Read the model definition and answer for the solid it produces. Units are mm, in the model's axes. Coordinates: 2 decimals unless noted, no trailing zeros. Write each loop counter-clockwise with the first axis right and the second up, starting at its lowest first coordinate (ties: lowest second). Pieces come first, ordered by that corner, then holes.
(1) The part is cut by section A-A, the plane x = -70. Determine the outline of the cut face in (y, z), and give its area (3 significant figures).
(2) Given pin 1 (9.5 mm diameter, centred on x = 0.5, y = 17, fed in from -Z); pin 2 (4 mm diameter, centred on y = 26, z = -8.5, fed in from -X); pin 3 (3.5 mm diameter, centred on x = -344.5, y = 13.5, fed in from -Z); pin 4 (5 mm diameter, centred on y = 12, z = 22.5, fed in from +X), each flat-ended and moving along its own axis, determine where each tip first touches the part or whether it passes through.
(3) Straight lines are drawn through the part: line 1 along X through (y, z) = (15, -12.5); line 2 along X through (y, z) = (15, -14); line 3 along Y through (x, z) = (345, -17). For each, find the intervals that lie inside material, in ascending order.
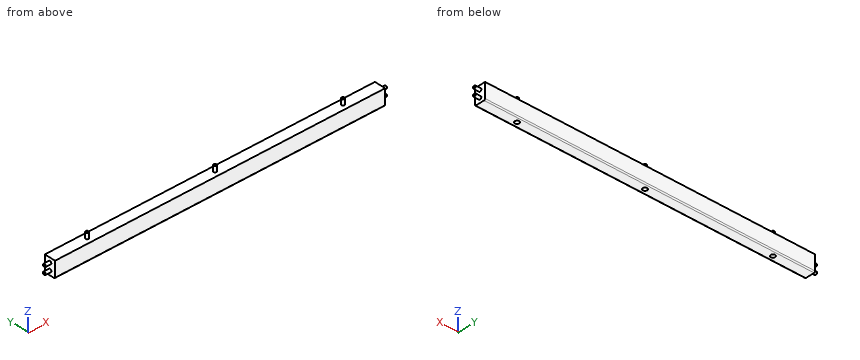
```python
from build123d import *

# Parameters (mm, degrees)
F0_W      = 890
F0_H      = 43
F1_DEPTH  = 30
F2_R      = 4
F3_DEPTH  = 16
F4_SIZE   = 1
F5_R      = 4
F6_DEPTH  = 16
F7_SIZE   = 1
F8_R      = 3
F9_R      = 6
F10_DEPTH = 16
F11_R     = 4
F12_DEPTH = 16
F13_SIZE  = 1


with BuildPart() as f1:
    # F0 (on Front) → F1 (new body)
    with BuildSketch(Plane.XZ):
        Rectangle(F0_W, F0_H)
    extrude(amount=-F1_DEPTH)

    # F2 (on face) → F3 (join)
    with BuildSketch(Plane.YZ.offset(445)):
        with Locations((15, 9.5)):
            Circle(F2_R)
        with Locations((15, -9.5)):
            Circle(F2_R)
    extrude(amount=F3_DEPTH)

    # F4
    f4_edges = [f1.edges().sort_by_distance(p)[0] for p in [
        (461, 11, 9.5),
        (461, 11, -9.5),
    ]]
    chamfer(f4_edges, length=F4_SIZE)

    # F5 (on face) → F6 (join)
    with BuildSketch(Plane(origin=(-445, 0, 0), x_dir=(0, -1, 0), z_dir=(-1, 0, 0))):
        with Locations((-15, 9.5)):
            Circle(F5_R)
        with Locations((-15, -9.5)):
            Circle(F5_R)
    extrude(amount=F6_DEPTH)

    # F7
    f7_edges = [f1.edges().sort_by_distance(p)[0] for p in [
        (-461, 19, 9.5),
        (-461, 19, -9.5),
    ]]
    chamfer(f7_edges, length=F7_SIZE)

    # F8
    f8_edges = [f1.edges().sort_by_distance(p)[0] for p in [
        (0, 30, -21.5),
        (0, 0, -21.5),
    ]]
    fillet(f8_edges, radius=F8_R)

    # F9 (on face) → F10 (cut)
    with BuildSketch(Plane(origin=(0, 0, -21.5), x_dir=(1, 0, 0), z_dir=(0, 0, -1))):
        with Locations((-345, -15)):
            Circle(F9_R)
        with Locations((0, -15)):
            Circle(F9_R)
        with Locations((345, -15)):
            Circle(F9_R)
    extrude(amount=-F10_DEPTH, mode=Mode.SUBTRACT)

    # F11 (on face) → F12 (join)
    with BuildSketch(Plane.XY.offset(21.5)):
        with Locations((0, 15)):
            Circle(F11_R)
        with Locations((-345, 15)):
            Circle(F11_R)
        with Locations((345, 15)):
            Circle(F11_R)
    extrude(amount=F12_DEPTH)

    # F13
    f13_edges = [f1.edges().sort_by_distance(p)[0] for p in [
        (-349, 15, 37.5),
        (-4, 15, 37.5),
        (341, 15, 37.5),
    ]]
    chamfer(f13_edges, length=F13_SIZE)


solid = f1.part
```
Computed:
1. outline: (0, -18.5) arc R3 ccw to (3, -21.5) - (27, -21.5) arc R3 ccw to (30, -18.5) - (30, 21.5) - (0, 21.5) - close
1. area: 1,290 mm2
2. pin 1: stops at z = -21.5
2. pin 2: stops at x = -445
2. pin 3: stops at z = -5.5
2. pin 4: stops at x = 445
3. line 1: x = -461 to -351, -339 to -6, 6 to 339, 351 to 461
3. line 2: x = -445 to -351, -339 to -6, 6 to 339, 351 to 445
3. line 3: y = 0 to 9, 21 to 30
